Verification items for this drawing (mm, ordinates from the low corner). Give positions to 0.01 mm unless a question says otherwise; leave off trailing zeros. Order: outer loops, then holes, each group sorted by start corner. A loop starts at its lowest first (then second) coordinate and runs counter-clockwise, first axis right, second up.
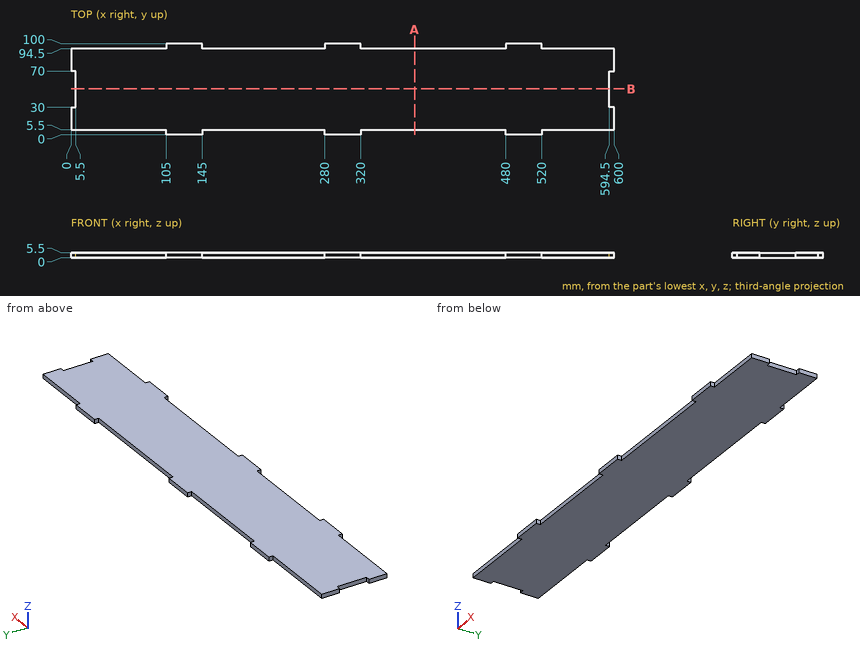
Q1. Cross-section at A-A, the plane x = 379.5. Record the boundary of the cut face in (y, z), and give its area (4 significant figures).
Q2. Gauge pin test, flat ends, axial feed: P1, Ø1.6, axis at y = 51.5, z = 1.5, coming from the +X side; P2, Ø3, axis at y = 98.5, z = 3, coming from the -X side; P3, Ø3, axis at x = 550.5, z = 3, coming from the -Y side. Record the tip position at first contact, or that the pin passes through.
Q3. Thickness scan on L1, parallel to Y at x = 58, z = 3.75; L2, parallel to X at y = 35.5, z = 0.8. Record the ranges inside material, lowest first.
Q4. Cross-section at B-B, the plane y = 50.5. Record the boundary of the cut face in (x, z), and give its area (3 significant figures).
Answers follow:
1. outline: (5.5, 0) - (94.5, 0) - (94.5, 5.5) - (5.5, 5.5) - close
1. area: 489.5 mm2
2. P1: stops at x = 594.5
2. P2: stops at x = 105
2. P3: stops at y = 5.5
3. L1: y = 5.5 to 94.5
3. L2: x = 5.5 to 594.5
4. outline: (5.5, 0) - (594.5, 0) - (594.5, 5.5) - (5.5, 5.5) - close
4. area: 3,240 mm2
